Geometry check sheet. Reference: the model listing, model coordinates, mm. Round coordinates to 2 decimals unless told otherwise and drop trailing zeros. Write each loop counter-clockwise with the first axis right and the second up, starting at its lowest first coordinate (ties: lowest second). Pieces come first, ordered by that corner, then holes. Notation, with made-up numbers: (20.25, 66) - (24.25, 66) arc R30 ccw to (24.25, 89) - close; hole circle Ø10 at (-3, 18.25). An arc over 180 degrees is marked (long way). Return JSON: item names as keys, results as strings.
```python
from build123d import *

# Parameters (mm, degrees)
SKETCH1_R           = 22.225
SKETCH1_R_2         = 19.05
BOSS_EXTRUDE1_DEPTH = 160
BOSS_EXTRUDE2_START = -160
SKETCH3_R           = 22.225
SKETCH3_R_2         = 6.35
BOSS_EXTRUDE2_DEPTH = 2.4
SKETCH4_R           = 7.55
SKETCH4_R_2         = 6.35
BOSS_EXTRUDE3_DEPTH = 10
FILLET1_SIZE        = 10
FILLET1_SIZE_2      = 5


with BuildPart() as part:
    # Sketch1 → Boss-Extrude1 (new body)
    with BuildSketch(Plane(origin=(0, 0, 0), x_dir=(1, 0, 0), z_dir=(0, 1, 0))):
        with Locations(Location((0, 0, 0), (0, 0, 270))):
            Circle(SKETCH1_R)
        with Locations(Location((0, 0, 0), (0, 0, 270))):
            Circle(SKETCH1_R_2, mode=Mode.SUBTRACT)
    extrude(amount=BOSS_EXTRUDE1_DEPTH)

    # Sketch3 → Boss-Extrude2 (add)
    with BuildSketch(Plane.XZ.offset(BOSS_EXTRUDE2_START)):
        with Locations(Location((0, 0, 0), (0, 0, 90))):
            Circle(SKETCH3_R)
        with Locations(Location((0, 0, 0), (0, 0, 90))):
            Circle(SKETCH3_R_2, mode=Mode.SUBTRACT)
    extrude(amount=-BOSS_EXTRUDE2_DEPTH)

    # Sketch4 → Boss-Extrude3 (add)
    with BuildSketch(Plane(origin=(0, 162.4, 0), x_dir=(-1, 0, 0), z_dir=(0, 1, 0))):
        with Locations(Location((0, 0, 0), (0, 0, 90))):
            Circle(SKETCH4_R)
        with Locations(Location((0, 0, 0), (0, 0, 90))):
            Circle(SKETCH4_R_2, mode=Mode.SUBTRACT)
    extrude(amount=BOSS_EXTRUDE3_DEPTH)

    # Fillet1
    # an asymmetric fillet: 10, 5 mm, written as the material it adds along each edge
    with BuildSketch(Plane(origin=(0, 162.4, 0), x_dir=(0, 0, 1), z_dir=(-1, 0, 0))) as fillet1_piece_1:
        with BuildLine():
            Bezier((7.55 + FILLET1_SIZE, 0), (7.55, 0), (7.55, FILLET1_SIZE_2), weights=[1, 0.707106781, 1])
            Line((7.55, FILLET1_SIZE_2), (7.55, 0))
            Line((7.55, 0), (7.55 + FILLET1_SIZE, 0))
        make_face()
    revolve(axis=Axis((0, 162.4, 0), (0, 1, 0)))


solid = part.part
```
(1) Section check A-A, the plane y = 82. Enter the section's corners in (x, z) (3 decimals), plus the area to 3 significant figures.
Response values:
{"outline": "circle Ø44.45 at (0, 0); hole circle Ø38.1 at (0, 0)", "area": "412 mm^2"}
(2) Material ranges on line 1 along X through (y, z) = (41.5, 0) (3 decimals); line 2 along X through (y, z) = (169.5, 0); line 3 along Z through (x, y) = (1, 124), recorded low to high. Write a range as [from, to].
Response values:
{"line 1": "x = [-22.225, -19.05], [19.05, 22.225]", "line 2": "x = [-7.55, -6.35], [6.35, 7.55]", "line 3": "z = [-22.2, -19.02], [19.02, 22.2]"}
(3) Release check for a two-part mould opening along X. For faces 1 (the face through (-5, 160, -5)), 2 (the face through (-6.7, 162.4, 16.4)), 3 (the face through (-7.37, 169.86, -1.64)), 4 (the face through (-11.59, 78.88, -15.12)) record: pulls with the +X half, pulls with the -X half, needs draft (parallel to the pull), parting line crosses it, or undercut.
Response values:
{"face 1": "undercut", "face 2": "needs draft", "face 3": "parting line crosses it", "face 4": "undercut"}
(4) Gauge pin test, flat ends, axial feed: pin 1 (1 mm diameter, centred on y = 123.5, z = 4.5, fed in from -X); pin 2 (2 mm diameter, centred on x = 6.5, z = 7.5, fed in from -Y); pin 3 (1.5 mm diameter, centred on x = -7, y = 146.5, fed in from +Z). Record the tip position at first contact, or that the pin passes through.
Response values:
{"pin 1": "stops at x = -21.86", "pin 2": "stops at y = 160", "pin 3": "stops at z = 21.33"}
